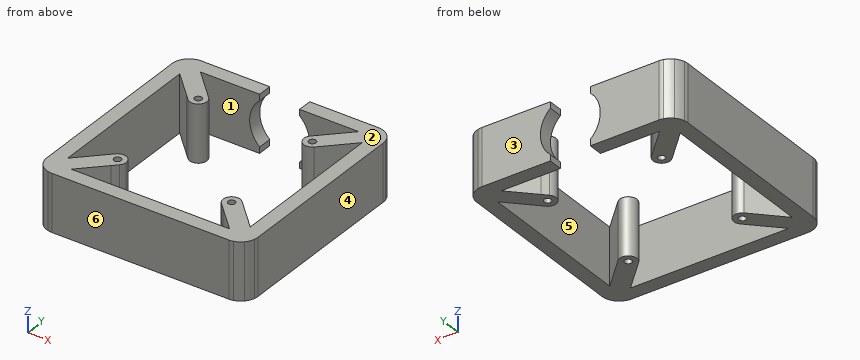
from build123d import *

# Parameters (mm, degrees)
F1_DEPTH = 20
F3_DEPTH = 25
F6_D     = 2.5


# Not quite as in the source:
# - a feature names something its author has since deleted; it is built from what else it names


with BuildPart() as f1:
    # F0 (on Top) → F1 (new body)
    with BuildSketch(Plane.XY):
        with BuildLine():
            Line((0, 68), (0, 6))
            ThreePointArc((0, 6), (0.0513308318, 5.2168428467), (0.2044450423, 4.4470857294))
            Line((0.2044450423, 4.4470857294), (5, 9.2426406871))
            Line((5, 9.2426406871), (5, 24.5))
            Line((5, 24.5), (5, 49))
            Line((5, 49), (5, 64.7573593129))
            Line((5, 64.7573593129), (0.2044450423, 69.5529142706))
            ThreePointArc((0.2044450423, 69.5529142706), (0.0513308318, 68.7831571533), (0, 68))
        make_face()
        with BuildLine():
            Line((5, 9.2426406871), (0.2044450423, 4.4470857294))
            ThreePointArc((0.2044450423, 4.4470857294), (0.8038475773, 3), (1.7573593129, 1.7573593129))
            Line((1.7573593129, 1.7573593129), (5.2928932188, 5.2928932188))
            ThreePointArc((5.2928932188, 5.2928932188), (5.0761204675, 5.6173165676), (5, 6))
            Line((5, 6), (5, 9.2426406871))
        make_face()
        with BuildLine():
            ThreePointArc((1.7573593129, 72.2426406871), (0.8038475773, 71), (0.2044450423, 69.5529142706))
            Line((0.2044450423, 69.5529142706), (5, 64.7573593129))
            Line((5, 64.7573593129), (5, 68))
            ThreePointArc((5, 68), (5.0761204675, 68.3826834324), (5.2928932188, 68.7071067812))
            Line((5.2928932188, 68.7071067812), (1.7573593129, 72.2426406871))
        make_face()
        with BuildLine():
            Line((5.2928932188, 5.2928932188), (1.7573593129, 1.7573593129))
            ThreePointArc((1.7573593129, 1.7573593129), (3, 0.8038475773), (4.4470857294, 0.2044450423))
            Line((4.4470857294, 0.2044450423), (9.2426406871, 5))
            Line((9.2426406871, 5), (6, 5))
            ThreePointArc((6, 5), (5.6173165676, 5.0761204675), (5.2928932188, 5.2928932188))
        make_face()
        with BuildLine():
            Line((14.8786796564, 19.1213203436), (5, 9.2426406871))
            Line((5, 9.2426406871), (5, 6))
            ThreePointArc((5, 6), (5.0761204675, 5.6173165676), (5.2928932188, 5.2928932188))
            Line((5.2928932188, 5.2928932188), (14.8786796564, 14.8786796564))
            ThreePointArc((14.8786796564, 14.8786796564), (14, 17), (14.8786796564, 19.1213203436))
        make_face()
        with BuildLine():
            ThreePointArc((4.4470857294, 73.7955549577), (3, 73.1961524227), (1.7573593129, 72.2426406871))
            Line((1.7573593129, 72.2426406871), (5.2928932188, 68.7071067812))
            ThreePointArc((5.2928932188, 68.7071067812), (5.6173165676, 68.9238795325), (6, 69))
            Line((6, 69), (9.2426406871, 69))
            Line((9.2426406871, 69), (4.4470857294, 73.7955549577))
        make_face()
        with BuildLine():
            Line((5, 68), (5, 64.7573593129))
            Line((5, 64.7573593129), (13.1819805153, 56.5753787975))
            Line((13.1819805153, 56.5753787975), (14.8786796564, 54.8786796564))
            ThreePointArc((14.8786796564, 54.8786796564), (14, 57), (14.8786796564, 59.1213203436))
            Line((14.8786796564, 59.1213203436), (5.2928932188, 68.7071067812))
            ThreePointArc((5.2928932188, 68.7071067812), (5.0761204675, 68.3826834324), (5, 68))
        make_face()
        with BuildLine():
            Line((9.2426406871, 5), (4.4470857294, 0.2044450423))
            ThreePointArc((4.4470857294, 0.2044450423), (5.2168428467, 0.0513308318), (6, 0))
            Line((6, 0), (37, 0))
            Line((37, 0), (68, 0))
            ThreePointArc((68, 0), (68.7831571533, 0.0513308318), (69.5529142706, 0.2044450423))
            Line((69.5529142706, 0.2044450423), (64.7573593129, 5))
            Line((64.7573593129, 5), (37, 5))
            Line((37, 5), (30, 5))
            Line((30, 5), (9.2426406871, 5))
        make_face()
        with BuildLine():
            Line((14.8786796564, 14.8786796564), (5.2928932188, 5.2928932188))
            ThreePointArc((5.2928932188, 5.2928932188), (5.6173165676, 5.0761204675), (6, 5))
            Line((6, 5), (9.2426406871, 5))
            Line((9.2426406871, 5), (17.4246212025, 13.1819805153))
            Line((17.4246212025, 13.1819805153), (19.1213203436, 14.8786796564))
            ThreePointArc((19.1213203436, 14.8786796564), (17, 14), (14.8786796564, 14.8786796564))
        make_face()
        with BuildLine():
            ThreePointArc((20, 17), (18.1480502971, 19.7716385975), (14.8786796564, 19.1213203436))
            ThreePointArc((14.8786796564, 19.1213203436), (14, 17), (14.8786796564, 14.8786796564))
            ThreePointArc((14.8786796564, 14.8786796564), (17, 14), (19.1213203436, 14.8786796564))
            ThreePointArc((19.1213203436, 14.8786796564), (19.7716385975, 15.8519497029), (20, 17))
        make_face()
        with BuildLine():
            ThreePointArc((6, 74), (5.2168428467, 73.9486691682), (4.4470857294, 73.7955549577))
            Line((4.4470857294, 73.7955549577), (9.2426406871, 69))
            Line((9.2426406871, 69), (30, 69))
            Line((30, 69), (30, 74))
            Line((30, 74), (6, 74))
        make_face()
        with BuildLine():
            ThreePointArc((6, 69), (5.6173165676, 68.9238795325), (5.2928932188, 68.7071067812))
            Line((5.2928932188, 68.7071067812), (14.8786796564, 59.1213203436))
            ThreePointArc((14.8786796564, 59.1213203436), (17, 60), (19.1213203436, 59.1213203436))
            Line((19.1213203436, 59.1213203436), (17.4246212025, 60.8180194847))
            Line((17.4246212025, 60.8180194847), (9.2426406871, 69))
            Line((9.2426406871, 69), (6, 69))
        make_face()
        with BuildLine():
            ThreePointArc((19.1213203436, 59.1213203436), (17, 60), (14.8786796564, 59.1213203436))
            ThreePointArc((14.8786796564, 59.1213203436), (14, 57), (14.8786796564, 54.8786796564))
            ThreePointArc((14.8786796564, 54.8786796564), (18.1480502971, 54.2283614025), (20, 57))
            ThreePointArc((20, 57), (19.7716385975, 58.1480502971), (19.1213203436, 59.1213203436))
        make_face()
        with BuildLine():
            Line((64.7573593129, 5), (69.5529142706, 0.2044450423))
            ThreePointArc((69.5529142706, 0.2044450423), (71, 0.8038475773), (72.2426406871, 1.7573593129))
            Line((72.2426406871, 1.7573593129), (68.7071067812, 5.2928932188))
            ThreePointArc((68.7071067812, 5.2928932188), (68.3826834324, 5.0761204675), (68, 5))
            Line((68, 5), (64.7573593129, 5))
        make_face()
        with BuildLine():
            Line((56.5753787975, 13.1819805153), (64.7573593129, 5))
            Line((64.7573593129, 5), (68, 5))
            ThreePointArc((68, 5), (68.3826834324, 5.0761204675), (68.7071067812, 5.2928932188))
            Line((68.7071067812, 5.2928932188), (59.1213203436, 14.8786796564))
            ThreePointArc((59.1213203436, 14.8786796564), (57, 14), (54.8786796564, 14.8786796564))
            Line((54.8786796564, 14.8786796564), (56.5753787975, 13.1819805153))
        make_face()
        with BuildLine():
            Line((68.7071067812, 5.2928932188), (72.2426406871, 1.7573593129))
            ThreePointArc((72.2426406871, 1.7573593129), (73.1961524227, 3), (73.7955549577, 4.4470857294))
            Line((73.7955549577, 4.4470857294), (69, 9.2426406871))
            Line((69, 9.2426406871), (69, 6))
            ThreePointArc((69, 6), (68.9238795325, 5.6173165676), (68.7071067812, 5.2928932188))
        make_face()
        with BuildLine():
            Line((69, 9.2426406871), (73.7955549577, 4.4470857294))
            ThreePointArc((73.7955549577, 4.4470857294), (73.9486691682, 5.2168428467), (74, 6))
            Line((74, 6), (74, 68))
            ThreePointArc((74, 68), (73.9486691682, 68.7831571533), (73.7955549577, 69.5529142706))
            Line((73.7955549577, 69.5529142706), (69, 64.7573593129))
            Line((69, 64.7573593129), (69, 49))
            Line((69, 49), (69, 24.5))
            Line((69, 24.5), (69, 9.2426406871))
        make_face()
        with BuildLine():
            Line((59.1213203436, 14.8786796564), (68.7071067812, 5.2928932188))
            ThreePointArc((68.7071067812, 5.2928932188), (68.9238795325, 5.6173165676), (69, 6))
            Line((69, 6), (69, 9.2426406871))
            Line((69, 9.2426406871), (59.1213203436, 19.1213203436))
            ThreePointArc((59.1213203436, 19.1213203436), (59.7716385975, 18.1480502971), (60, 17))
            ThreePointArc((60, 17), (59.7716385975, 15.8519497029), (59.1213203436, 14.8786796564))
        make_face()
        with BuildLine():
            ThreePointArc((59.1213203436, 19.1213203436), (54.8786796564, 19.1213203436), (54.8786796564, 14.8786796564))
            ThreePointArc((54.8786796564, 14.8786796564), (57, 14), (59.1213203436, 14.8786796564))
            ThreePointArc((59.1213203436, 14.8786796564), (59.7716385975, 15.8519497029), (60, 17))
            ThreePointArc((60, 17), (59.7716385975, 18.1480502971), (59.1213203436, 19.1213203436))
        make_face()
        with BuildLine():
            Line((69, 64.7573593129), (73.7955549577, 69.5529142706))
            ThreePointArc((73.7955549577, 69.5529142706), (73.1961524227, 71), (72.2426406871, 72.2426406871))
            Line((72.2426406871, 72.2426406871), (68.7071067812, 68.7071067812))
            ThreePointArc((68.7071067812, 68.7071067812), (68.9238795325, 68.3826834324), (69, 68))
            Line((69, 68), (69, 64.7573593129))
        make_face()
        with BuildLine():
            Line((68.7071067812, 68.7071067812), (72.2426406871, 72.2426406871))
            ThreePointArc((72.2426406871, 72.2426406871), (71, 73.1961524227), (69.5529142706, 73.7955549577))
            Line((69.5529142706, 73.7955549577), (64.7573593129, 69))
            Line((64.7573593129, 69), (68, 69))
            ThreePointArc((68, 69), (68.3826834324, 68.9238795325), (68.7071067812, 68.7071067812))
        make_face()
        with BuildLine():
            Line((59.1213203436, 54.8786796564), (69, 64.7573593129))
            Line((69, 64.7573593129), (69, 68))
            ThreePointArc((69, 68), (68.9238795325, 68.3826834324), (68.7071067812, 68.7071067812))
            Line((68.7071067812, 68.7071067812), (59.1213203436, 59.1213203436))
            ThreePointArc((59.1213203436, 59.1213203436), (59.7716385975, 58.1480502971), (60, 57))
            ThreePointArc((60, 57), (59.7716385975, 55.8519497029), (59.1213203436, 54.8786796564))
        make_face()
        with BuildLine():
            Line((64.7573593129, 69), (69.5529142706, 73.7955549577))
            ThreePointArc((69.5529142706, 73.7955549577), (68.7831571533, 73.9486691682), (68, 74))
            Line((68, 74), (44, 74))
            Line((44, 74), (44, 69))
            Line((44, 69), (64.7573593129, 69))
        make_face()
        with BuildLine():
            Line((59.1213203436, 59.1213203436), (68.7071067812, 68.7071067812))
            ThreePointArc((68.7071067812, 68.7071067812), (68.3826834324, 68.9238795325), (68, 69))
            Line((68, 69), (64.7573593129, 69))
            Line((64.7573593129, 69), (56.5753787975, 60.8180194847))
            Line((56.5753787975, 60.8180194847), (54.8786796564, 59.1213203436))
            ThreePointArc((54.8786796564, 59.1213203436), (57, 60), (59.1213203436, 59.1213203436))
        make_face()
        with BuildLine():
            ThreePointArc((54.8786796564, 59.1213203436), (54.8786796564, 54.8786796564), (59.1213203436, 54.8786796564))
            ThreePointArc((59.1213203436, 54.8786796564), (59.7716385975, 55.8519497029), (60, 57))
            ThreePointArc((60, 57), (59.7716385975, 58.1480502971), (59.1213203436, 59.1213203436))
            ThreePointArc((59.1213203436, 59.1213203436), (57, 60), (54.8786796564, 59.1213203436))
        make_face()
    extrude(amount=F1_DEPTH)


with BuildPart() as f3:
    # F2 (on face) → F3 (new body)
    with BuildSketch(Plane(origin=(0, 74, 0), x_dir=(-1, 0, 0), z_dir=(0, 1, 0))):
        with BuildLine():
            ThreePointArc((-26.5, 10), (-37, 20.5), (-47.5, 10))
            Line((-47.5, 10), (-26.5, 10))
        make_face()
        with BuildLine():
            Line((-26.5, 10), (-47.5, 10))
            ThreePointArc((-47.5, 10), (-37, -0.5), (-26.5, 10))
        make_face()
    extrude(amount=-F3_DEPTH)


with BuildPart() as f1_1:
    add(f1.part)

    # F4: cut F3
    add(f3.part, mode=Mode.SUBTRACT)

    # F6 (through all)
    with Locations(Plane.XY.offset(20)):
        with Locations((17, 57), (57, 57), (57, 17), (17, 17)):
            Hole(F6_D / 2)


solid = f1_1.part
Verification items for the finished model (mm, model axes). Face numbers are marked on the shaded views. A direction names the side the tool comes from. Give positions to 0.01 mm unless a question says otherwise; leave off trailing zeros. Loops run counter-clockwise (first coordinate to the right, second up) from the corner with the lowest first, then second, coordinate; pieces in that order, holes last.
1) Depth check by flat-ended pin: pin 1 Ø2.5 at (y, z) = (72, 1) entering from +X; pin 2 Ø1.7 at (y, z) = (71, 19) entering from -X; pin 3 Ø0.7 at (y, z) = (70.5, 19.5) entering from +X. Enter the tip coordinate at first touch or a pass-through.
2) Sectioned sample at A-A, the plane y = 37.5. Enter the section's corners in (x, z), then the cut area to 3 significant figures.
3) Sectioned sample at D-D, the plane z = 15.25. Count the separate pieces of the cut face and the enclosed holes in it, then the cut area to 3 significant figures.
4) Thickness scan on line 1 along X through (y, z) = (49.5, 1); line 2 along Y through (x, z) = (63, 4.75); line 3 along Y through (x, z) = (14, 18.5). Record the ranges inside material, lowest first.
5) Draft check along Y on the marked faces 3, 4, 5 and 6. Enter one of: pulls with the +Y half, pulls with the -Y half, needs draft (parallel to the pull), parting line crosses it, or undercut.
6) Set-up check for the marked faces 1 and 2: record each of +Z, -Z, +X, -X, +Y, -Y from which the full face is reachable in a straight line by a thin tool's end or side.
7) Sectioned sample at C-C, the plane y = 62.5. Enter the section's corners in (x, z).
Answers:
1. pin 1: stops at x = 73.33
1. pin 2: stops at x = 0.4
1. pin 3: stops at x = 73.6
2. outline: (0, 0) - (5, 0) - (5, 20) - (0, 20) - close; (69, 0) - (74, 0) - (74, 20) - (69, 20) - close
2. area: 200 mm2
3. separate pieces: 1
3. enclosed holes: 4
3. area: 1,670 mm2
4. line 1: x = 0 to 5, 69 to 74
4. line 2: y = 0 to 5, 6.76 to 15.24, 58.76 to 67.24, 69 to 74
4. line 3: y = 0 to 5, 9.76 to 18.24, 55.76 to 64.24, 69 to 74
5. face 3: pulls with the +Y half
5. face 4: needs draft
5. face 5: undercut
5. face 6: pulls with the -Y half
6. face 1: +Z, -Z
6. face 2: +Z, +X, -X, +Y, -Y
7. outline: (0, 0) - (5, 0) - (5, 20) - (0, 20) - close; (7.26, 0) - (15.74, 0) - (15.74, 20) - (7.26, 20) - close; (58.26, 0) - (66.74, 0) - (66.74, 20) - (58.26, 20) - close; (69, 0) - (74, 0) - (74, 20) - (69, 20) - close
